Verification items for this drawing (mm, ordinates from the low corner). A direction names the side the tool comes from. Give positions to 0.01 mm unless a question says otherwise; leave off trailing zeros. Order: outer loops, then holes, each group sorted by start corner. A loop starts at its lowest first (then second) coordinate and runs counter-clockwise, first axis right, second up.
(1) Gauge pin test, flat ends, axial feed: pin 1 (1 mm diameter, centred on y = 9.5, z = 51.5, fed in from -X); pin 2 (8 mm diameter, centred on y = 4, z = 27.5, fed in from -X); pin 3 (1 mm diameter, centred on x = 59, y = 19, fed in from +Z). Record the tip position at first contact, or that the pin passes through.
(2) Access from +Z, -Z, +X, -X, +Y, -Y to the whole of each face (thin tool, end or side, straight path). Record for the marked faces 1 and 2.
(3) Mould release check, pull along Z, two halves, no side actions. Record for the marked faces 3, 4, 5 and 6: pulls with the +Z half, pulls with the -Z half, needs draft (parallel to the pull), parting line crosses it, or undercut.
(4) Sectioned sample at C-C on y = 15. Record the cut outline in (x, z), plus the area to 3 significant figures.
(5) Sectioned sample at A-A on x = 30.5. Record the cut outline in (y, z) (1 decimal), plus the area to 3 significant figures.
(6) Scan lines: L1, parallel to X at y = 23.75, z = 36 (1 decimal); L2, parallel to Z at x = 46, y = 22 (1 decimal); L3, parallel to X at y = 25.25, z = 65.5 (1 decimal). Record each from-to range of solid material in increasing order.
(7) Sectioned sample at D-D on x = 71. Record the cut outline in (y, z) (1 decimal).
(8) Sectioned sample at B-B on y = 25. Record the cut outline in (x, z).
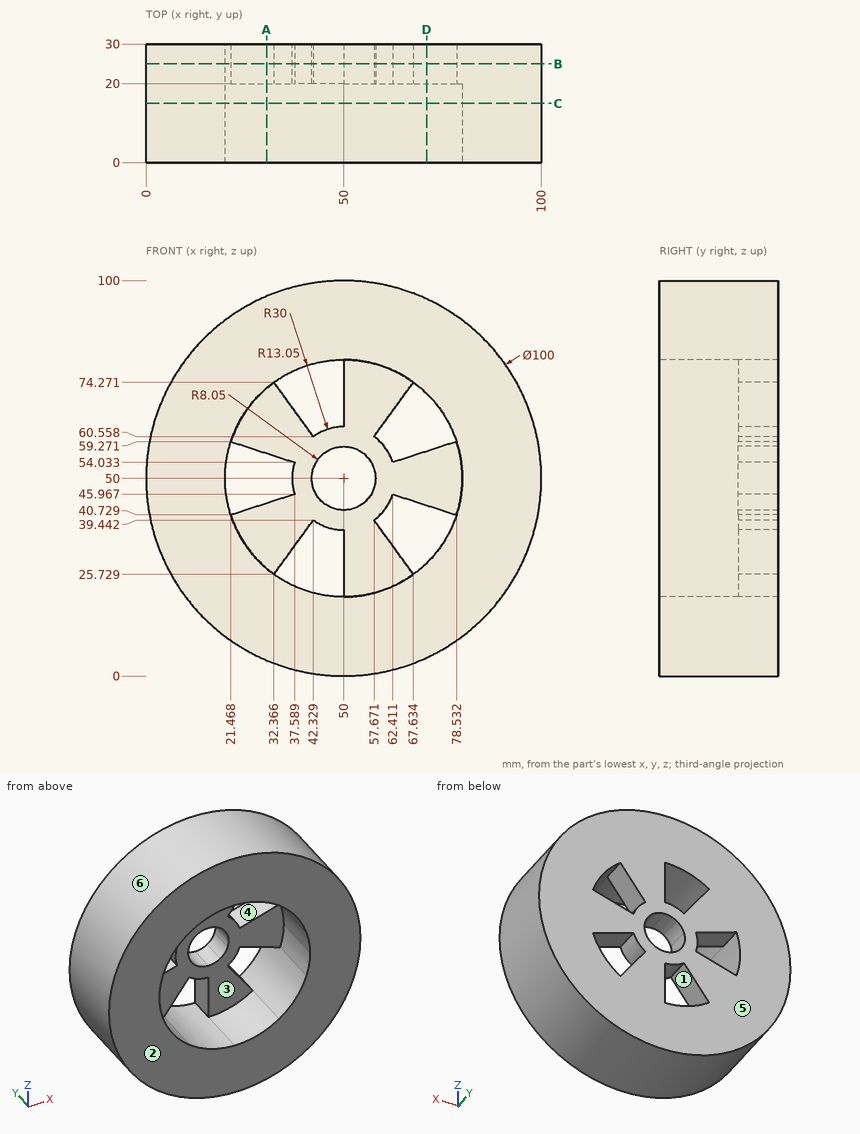
Ans:
1. pin 1: stops at x = 0.01
1. pin 2: stops at x = 3.55
1. pin 3: stops at z = 99.27
2. face 1: +Y, -Y
2. face 2: +Z, -Z, +X, -X, -Y
3. face 3: undercut
3. face 4: undercut
3. face 5: needs draft
3. face 6: parting line crosses it
4. outline: circle Ø100 at (50, 50); hole circle Ø60 at (50, 50)
4. area: 5,030 mm2
5. outline: (0, 4) - (30, 4) - (30, 43.7) - (20, 43.7) - (20, 27.2) - (0, 27.2) - close; (0, 72.8) - (20, 72.8) - (20, 56.3) - (30, 56.3) - (30, 96) - (0, 96) - close
5. area: 1,720 mm2
6. L1: x = 2 to 39.8, 50 to 60.2, 76.5 to 98
6. L2: z = 0.2 to 20.3, 37.6 to 43, 57 to 62.4, 79.7 to 99.8
6. L3: x = 2.5 to 38.7, 50 to 61.3, 75.7 to 97.5
7. outline: (0, 4.6) - (30, 4.6) - (30, 28.6) - (0, 28.6) - close; (0, 71.4) - (30, 71.4) - (30, 95.4) - (0, 95.4) - close; (20, 43.2) - (30, 43.2) - (30, 56.8) - (20, 56.8) - close
8. outline: circle Ø100 at (50, 50); hole (21.47, 40.73) - (37.59, 45.97) arc R13.05 cw to (37.59, 54.03) - (21.47, 59.27) arc R30 ccw to start; hole (32.37, 25.73) arc R30 ccw to (50, 20) - (50, 36.95) arc R13.05 cw to (42.33, 39.44) - close; hole (32.37, 74.27) - (42.33, 60.56) arc R13.05 cw to (50, 63.05) - (50, 80) arc R30 ccw to start; hole circle Ø16.1 at (50, 50); hole (57.67, 39.44) - (67.63, 25.73) arc R30 ccw to (78.53, 40.73) - (62.41, 45.97) arc R13.05 cw to start; hole (57.67, 60.56) arc R13.05 cw to (62.41, 54.03) - (78.53, 59.27) arc R30 ccw to (67.63, 74.27) - close
